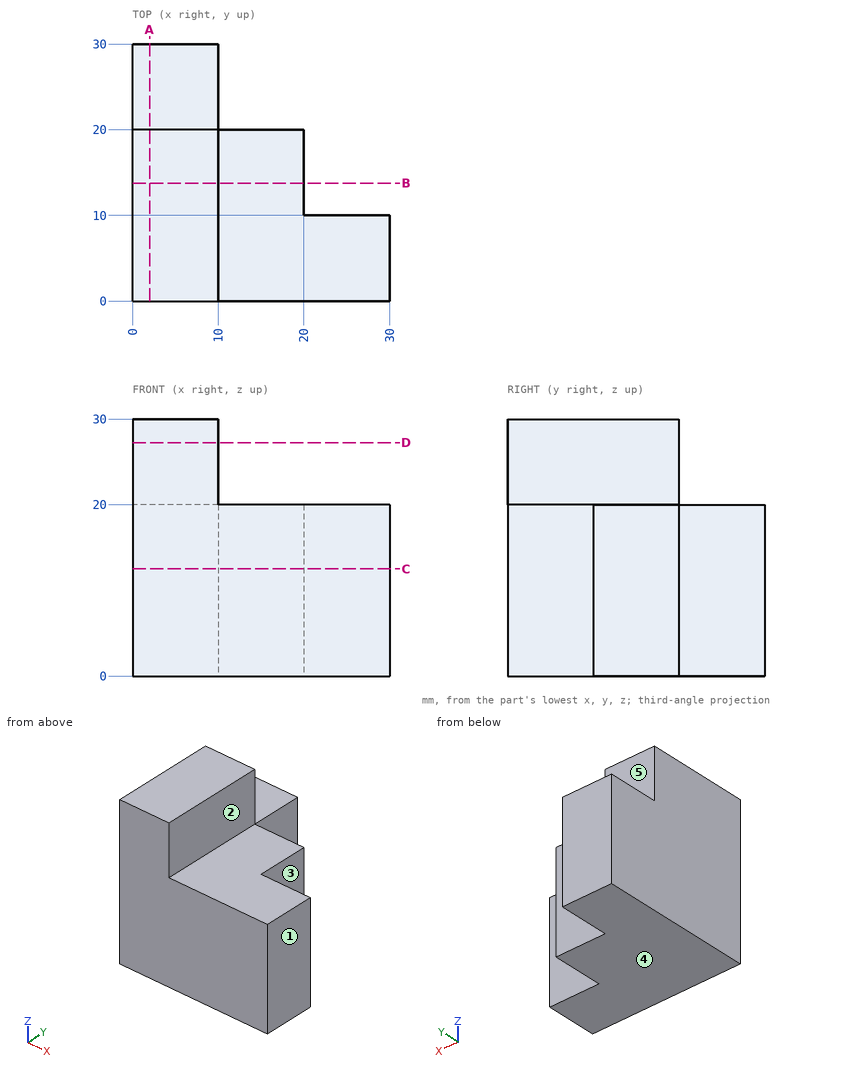
Verification items for this drawing (mm, ordinates from the low corner). A direction names the side the tool comes from. Give positions to 0.01 mm unless a question says otherwise; leave off trailing zeros. Write each loop counter-clockwise with the first axis right and the second up, starting at its lowest first coordinate (ties: lowest second). Pieces come first, ordered by that corner, then holes. Notation, with made-up numbers: M 72,-29 L 120,-29 A25 cw 120,-14 Z; hole C 87.5,28.5 d2. An arc over 180 degrees is marked long. Use one line per item in the form item = value.
(1) Material ranges on line 1 along Z through (x, y) = (7.5, 21.75); line 2 along X through (y, z) = (21, 4.5), recorded low to high.
Answer block:
line_1 = 0 to 20
line_2 = 0 to 10
(2) Section check D-D on z = 27.25. Record the boundary of the cut face in (x, y), plus the area to 3 significant figures.
Answer block:
outline = M 0,0 L 10,0 L 10,20 L 0,20 Z
area = 200 mm2
(3) Tool access check on the marked faces 1, 2, 3, 4 and 5. Record the directions out of +Z, -Z, +X, -X, +Y, -Y that give a thin tool (end or side, any length) a straight path to the whole face; none if there is none.
Answer block:
face_1 = +Z, -Z, +X, +Y, -Y
face_2 = +Z, +X, +Y, -Y
face_3 = +Z, -Z, +X, +Y
face_4 = -Z, +X, -X, +Y, -Y
face_5 = +Z, +X, -X, +Y
(4) Section check A-A on x = 2. Record the boundary of the cut face in (y, z), plus the area to 3 significant figures.
Answer block:
outline = M 0,0 L 30,0 L 30,20 L 20,20 L 20,30 L 0,30 Z
area = 800 mm2
(5) Section check B-B on y = 13.75. Record the boundary of the cut face in (x, z).
Answer block:
outline = M 0,0 L 20,0 L 20,20 L 10,20 L 10,30 L 0,30 Z
(6) Section check C-C on z = 12.5. Record the boundary of the cut face in (x, y), plus the area to 3 significant figures.
Answer block:
outline = M 0,0 L 30,0 L 30,10 L 20,10 L 20,20 L 10,20 L 10,30 L 0,30 Z
area = 600 mm2
(7) Depth check by flat-ended pin: P1, Ø4, axis at x = 16, z = 16.5, coming from the +Y side; P2, Ø3, axis at y = 8, z = 25, coming from the +X side; P3, Ø3, axis at x = 26, z = 8, coming from the +Y side; P4, Ø3, axis at x = 13, z = 22.5, coming from the +Y side. Enter the tip coordinate at first touch or a pass-through.
Answer block:
P1 = 20
P2 = 10
P3 = 10
P4 = through
